Part model, mm, in its own coordinate system. A direction names the side the tool comes from. Coordinates: 2 decimals unless noted, no trailing zeros. Write each loop counter-clockwise with the first axis right and the second up, starting at its lowest first coordinate (ties: lowest second). Pieces come first, ordered by that corner, then holes. Notation, with made-up numbers: (30.5, 34) -> (87.5, 34) arc R16 cw to (87.5, 46) -> close; hole circle Ø4 at (53, 59). An arc over 180 degrees is marked (long way). One line per question, with ' | ' between items. Start each with the question number.
Item 1: Saw through at D-D (y = -10.5). List the corners of the cut face in (x, z), and give its area (3 significant figures).
Item 2: Saw through at B-B (z = 1.8). List the corners of the cut face in (x, y).
Item 3: Saw through at A-A (y = 0). List the corners of the cut face in (x, z).
Item 4: 3-axis set-ups, long thin cutter, end or side, ignore diameter. For faces 1 (the flat face through (17.61, -8.42, 1.48)), 2 (the flat face through (157.49, 19.18, 1.48)): which of +Z, -Z, +X, -X, +Y, -Y reach the whole face in a straight line?
Item 5: Probe probe 1 along Y at (x, z) = (73.5, 0.6); probe 2 along X at (y, z) = (4, 1.95); probe 3 along Y at (x, z) = (127, 2.4). List the from-to ranges inside material, lowest first. Write a range as [from, to].
Item 6: Two-plate mould, pull along X, no slides. Class faces 3 (the cylindrical face through (-4.4, 8.98, 1.48)), 4 (the flat face through (111, -7, 3)), 5 (the flat face through (98.49, -5.25, 1.48)), 6 (the flat face through (-4.736, -15.615, 1.479)): pulls with the +X half, pulls with the -X half, needs draft (parallel to the pull), parting line crosses it, or undercut.
Item 7: Saw through at C-C (x = 131). List the corners of the cut face in (y, z), and give its area (3 significant figures).
Item 8: Pin check, flat tip, straight feed: pin 1 (1.5 mm diameter, centred on x = 46.5, z = 1, fed in from +Y). Stop position of the tip, or through.
from build123d import *

# Parameters (mm, degrees)
SKETCH_1_R      = 8
EXTRUDE_1_DEPTH = 3


with BuildPart() as part:
    # Эскиз1 → Бобышка-Вытянуть1 (new body)
    with BuildSketch(Plane.XY):
        with BuildLine():
            Line((-9.340497736, -3.571428571), (0, -28))
            Line((0, -28), (187.92551716, -28))
            ThreePointArc((187.92551716, -28), (189.991352408, -1.812735596), (188.425560886, 24.409178696))
            Line((188.425560886, 24.409178696), (125.667350293, 13.804301697))
            ThreePointArc((125.667350293, 13.804301697), (122.358795725, 12.813150055), (119.393575063, 11.042166898))
            Line((119.393575063, 11.042166898), (77, -22))
            Line((77, -22), (26.641557218, -22))
            Line((26.641557218, -22), (8.326583423, 5.537870395))
            ThreePointArc((8.326583423, 5.537870395), (-4.582776175, 8.888091051), (-9.340497736, -3.571428571))
        make_face()
        with Locations((128, 0)):
            Circle(SKETCH_1_R, mode=Mode.SUBTRACT)
    extrude(amount=EXTRUDE_1_DEPTH)


solid = part.part
From the geometry:
1) outline: (-6.69, 0) -> (18.99, 0) -> (18.99, 3) -> (-6.69, 3) -> close; (91.75, 0) -> (189.71, 0) -> (189.71, 3) -> (91.75, 3) -> close | area: 371 mm2
2) outline: (-9.34, -3.57) -> (0, -28) -> (187.93, -28) arc R190 ccw to (188.43, 24.41) -> (125.67, 13.8) arc R14 ccw to (119.39, 11.04) -> (77, -22) -> (26.64, -22) -> (8.33, 5.54) arc R10 ccw to start; hole circle Ø16 at (128, 0)
3) outline: (-10, 0) -> (12.01, 0) -> (12.01, 3) -> (-10, 3) -> close; (105.23, 0) -> (120, 0) -> (120, 3) -> (105.23, 3) -> close; (136, 0) -> (190, 0) -> (190, 3) -> (136, 3) -> close
4) face 1: +Z, -Z, +Y | face 2: +Z, -Z, -X, +Y
5) probe 1: [-28, -22] | probe 2: [-9.17, 9.35], [110.36, 121.07], [134.93, 189.96] | probe 3: [-28, -7.94], [7.94, 14.03]
6) face 3: undercut | face 4: needs draft | face 5: undercut | face 6: pulls with the -X half
7) outline: (-28, 0) -> (-7.42, 0) -> (-7.42, 3) -> (-28, 3) -> close; (7.42, 0) -> (14.71, 0) -> (14.71, 3) -> (7.42, 3) -> close | area: 83.6 mm2
8) pin 1: y = -22
